```python
from build123d import *

# Parameters (mm, degrees)
F0_W     = 171.45
F0_H     = 88.9
F1_DEPTH = 215.9
F2_W     = 40.64
F2_H     = 25.4
F2_W_2   = 27.94
F2_H_2   = 20.32
F2_W_3   = 10.16
F2_H_3   = 15.24
F3_DEPTH = 17.78
F4_W     = 81.28
F4_H     = 81.28
F4_R     = 9.525
F5_DEPTH = 25.4
F7_DEPTH = 1.524


with BuildPart() as f1:
    # F0 (on Front) → F1 (new body)
    with BuildSketch(Plane.XZ):
        with Locations((-85.725, 44.45)):
            Rectangle(F0_W, F0_H)
    extrude(amount=F1_DEPTH)

    # F2 (on face) → F3 (join)
    with BuildSketch(Plane.XZ.offset(215.9)):
        with Locations((-135.89, 17.78)):
            Rectangle(F2_W, F2_H)
        with Locations((-106.68, 64.77)):
            Rectangle(F2_W_2, F2_H_2)
        with Locations((-95.25, 20.32)):
            Rectangle(F2_W_3, F2_H_3)
    extrude(amount=F3_DEPTH)

    # F4 (on face) → F5 (join)
    with BuildSketch(Plane(origin=(0, 0, 0), x_dir=(-1, 0, 0), z_dir=(0, 1, 0))):
        with Locations((44.45, 44.45)):
            Rectangle(F4_W, F4_H)
        with Locations((151.13, 71.12)):
            Circle(F4_R)
    extrude(amount=F5_DEPTH)

    # F6 (on face) → F7 (join)
    with BuildSketch(Plane(origin=(0, 0, 0), x_dir=(1, 0, 0), z_dir=(0, 0, -1))):
        with BuildLine():
            Line((-184.15, 25.4), (-171.45, 25.4))
            Line((-171.45, 25.4), (-171.45, 82.55))
            Line((-171.45, 82.55), (-184.15, 82.55))
            Line((-184.15, 82.55), (-184.15, 57.785))
            Line((-184.15, 57.785), (-180.1876, 57.785))
            ThreePointArc((-180.1876, 57.785), (-176.3776, 53.975), (-180.1876, 50.165))
            Line((-180.1876, 50.165), (-184.15, 50.165))
            Line((-184.15, 50.165), (-184.15, 25.4))
        make_face()
        with BuildLine():
            Line((-184.15, 133.35), (-171.45, 133.35))
            Line((-171.45, 133.35), (-171.45, 190.5))
            Line((-171.45, 190.5), (-184.15, 190.5))
            Line((-184.15, 190.5), (-184.15, 165.735))
            Line((-184.15, 165.735), (-180.1876, 165.735))
            ThreePointArc((-180.1876, 165.735), (-176.3776, 161.925), (-180.1876, 158.115))
            Line((-180.1876, 158.115), (-184.15, 158.115))
            Line((-184.15, 158.115), (-184.15, 133.35))
        make_face()
        with BuildLine():
            Line((0, 190.5), (0, 133.35))
            Line((0, 133.35), (12.7, 133.35))
            Line((12.7, 133.35), (12.7, 158.115))
            Line((12.7, 158.115), (8.7376, 158.115))
            ThreePointArc((8.7376, 158.115), (4.9276, 161.925), (8.7376, 165.735))
            Line((8.7376, 165.735), (12.7, 165.735))
            Line((12.7, 165.735), (12.7, 190.5))
            Line((12.7, 190.5), (0, 190.5))
        make_face()
        with BuildLine():
            Line((0, 82.55), (0, 25.4))
            Line((0, 25.4), (12.7, 25.4))
            Line((12.7, 25.4), (12.7, 50.165))
            Line((12.7, 50.165), (8.7376, 50.165))
            ThreePointArc((8.7376, 50.165), (4.9276, 53.975), (8.7376, 57.785))
            Line((8.7376, 57.785), (12.7, 57.785))
            Line((12.7, 57.785), (12.7, 82.55))
            Line((12.7, 82.55), (0, 82.55))
        make_face()
    extrude(amount=-F7_DEPTH)


solid = f1.part
```
Check sheet for the modelled part. Datum: model origin and axes. Units: mm. A direction names the side the tool comes from. Give positions to 0.01 mm unless a question says otherwise; leave off trailing zeros. Write each loop counter-clockwise with the first axis right and the second up, starting at its lowest first coordinate (ties: lowest second). Pieces come first, ordered by that corner, then holes. Notation, with made-up numbers: (59, 45) - (96, 45) arc R8 ccw to (96, 54) - close; hole circle Ø1 at (-18.5, -13). An arc over 180 degrees is marked (long way). Answer as a JSON object with one key per item and string values. Group by question number.
1) Sectioned sample at D-D (x = -97.5). Record the cut outline in (y, z), then the cut area to 3 significant figures.
2) Release check for a two-part mould opening along X. For faces 1 (the face through (-136, -233.68, 18)), 2 (the face through (-125, 0, 45)), 3 (the face through (-100.33, -225, 20)), 4 (the face through (-90.17, -225, 20)) record: pulls with the +X half, pulls with the -X half, needs draft (parallel to the pull), parting line crosses it, or undercut.
3) Sectioned sample at B-B (x = -151.13). Record the cut outline in (y, z) (3 decimals), then the cut area to 3 significant figures.
4) Depth check by flat-ended pin: P1, Ø8, axis at x = -42, z = 10.5, coming from the -Y side; P2, Ø0.5, axis at x = 6.5, z = 0.5, coming from the -Y side; P3, Ø7.5, axis at y = -224, z = 21, coming from the -X side. Enter the tip coordinate at first touch or a pass-through.
5) Access from +Z, -Z, +X, -X, +Y, -Y to the whole of each face (thin tool, end or side, straight path). Record for faces 5 (the face through (-3.81, 13, 44)), 6 (the face through (-44, 13, 85.09)), 7 (the face through (-107, -225, 54.61)), 8 (the face through (-95, -225, 27.94)), 9 (the face through (3, -162, 1.524)).
6) Thickness scan on probe 1 along X at (y, z) = (-82, 60); probe 2 along Y at (x, z) = (-24.5, 61); probe 3 along Y at (x, z) = (-3.5, 39). Record the ranges inside material, lowest first. Write a range as from..to.
7) Sectioned sample at C-C (y = -42). Record the cut outline in (x, z), then the cut area to 3 significant figures.
8) Sectioned sample at A-A (z = 48). Record the cut outline in (x, y).
Geometry results:
{
 "1": {"outline": "(-233.68, 12.7) - (-215.9, 12.7) - (-215.9, 0) - (0, 0) - (0, 88.9) - (-215.9, 88.9) - (-215.9, 74.93) - (-233.68, 74.93) - (-233.68, 54.61) - (-215.9, 54.61) - (-215.9, 27.94) - (-233.68, 27.94) - close", "area": "19,800 mm^2"},
 "2": {"face 1": "needs draft", "face 2": "undercut", "face 3": "undercut", "face 4": "pulls with the +X half"},
 "3": {"outline": "(-233.68, 5.08) - (-215.9, 5.08) - (-215.9, 0) - (0, 0) - (0, 61.595) - (25.4, 61.595) - (25.4, 80.645) - (0, 80.645) - (0, 88.9) - (-215.9, 88.9) - (-215.9, 30.48) - (-233.68, 30.48) - close", "area": "20,100 mm^2"},
 "4": {"P1": "stops at y = -215.9", "P2": "stops at y = -190.5", "P3": "stops at x = -156.21"},
 "5": {"face 5": "+Z, -Z, +X, +Y", "face 6": "+Z, +X, -X, +Y", "face 7": "+X, -X, -Y", "face 8": "+X, -Y", "face 9": "+Z, +X, +Y, -Y"},
 "6": {"probe 1": "x = -171.45..0", "probe 2": "y = -215.9..25.4", "probe 3": "y = -215.9..0"},
 "7": {"outline": "(-184.15, 0) - (12.7, 0) - (12.7, 1.52) - (0, 1.52) - (0, 88.9) - (-171.45, 88.9) - (-171.45, 1.52) - (-184.15, 1.52) - close", "area": "15,300 mm^2"},
 "8": {"outline": "(-171.45, -215.9) - (0, -215.9) - (0, 0) - (-3.81, 0) - (-3.81, 25.4) - (-85.09, 25.4) - (-85.09, 0) - (-171.45, 0) - close"}
}
